Verification items for the finished model (mm, model axes). A direction names the side the tool comes from. Give positions to 0.01 mm unless a question says otherwise; leave off trailing zeros. Order: outer loops, then holes, each group sorted by start corner. A loop starts at its lowest first (then second) coordinate and runs counter-clockwise, first axis right, second up. Notation, with made-up numbers: (20.5, 48.25) - (69.5, 48.25) arc R21 ccw to (69.5, 61.25) - close; hole circle Ø1 at (-10, 52.5). An arc over 180 degrees is marked (long way). Answer as a JSON object with one key per item and string values. Group by question number.
(1) Section check B-B (x = -9.5). Record the boundary of the cut face in (y, z), then the cut area to 3 significant figures.
(2) Access from +Z, -Z, +X, -X, +Y, -Y to the whole of each face (thin tool, end or side, straight path). Record for faces 5 (the face through (-14, 2, 11)), 6 (the face through (-17.859, 62.797, 12.422)).
(3) Mould release check, pull along X, two halves, no side actions. Record for faces 1 (the face through (-1.203, 1.141, 12.422)), 2 (the face through (-5.87, 37.69, 23.51)), 3 (the face through (-19, 32, 12)), 4 (the face through (-8, 4, 0)): +X half, -X half, draft (parallel to the pull), parting line (faces both ways), or undercut.
(4) Section check D-D (y = 51). Record the boundary of the cut face in (x, z).
(5) Thickness scan on line 1 (Y direction, x = -9.5, z = 6.75); line 2 (X direction, y = 20.5, z = 2.5); line 3 (Y direction, x = -9.5, z = 23.3). Record the ranges inside material, lowest first.
(6) Section check A-A (y = 32). Record the boundary of the cut face in (x, z), then the cut area to 3 significant figures.
(7) Section check C-C (z = 20.75). Record the boundary of the cut face in (x, y), then the cut area to 3 significant figures.
```python
from build123d import *

# Parameters (mm, degrees)
F0_W      = 19
F0_H      = 64
F1_DEPTH  = 24.5
F3_DEPTH  = 25
F4_T      = -2
F5_R      = 4
F6_R      = 6.75
F7_DEPTH  = 25
F8_R      = 2
F8_R_2    = 1.25
F9_DEPTH  = 22.5
F10_R     = 6.75
F11_DEPTH = 25


with BuildPart() as f1:
    # F0 (on Top) → F1 (new body)
    with BuildSketch(Plane.XY):
        with Locations((-9.5, 32)):
            Rectangle(F0_W, F0_H)
    extrude(amount=F1_DEPTH)

    # F2 (on face) → F3 (cut)
    with BuildSketch(Plane.YZ):
        with BuildLine():
            Line((21, 0), (43, 0))
            ThreePointArc((43, 0), (32, 11), (21, 0))
        make_face()
    extrude(amount=-F3_DEPTH, mode=Mode.SUBTRACT)

    # F4
    f4_openings = [f1.faces().sort_by_distance(p)[0] for p in [
        (-9.5, 32, 11),
        (-9.5, 10.5, 0),
        (-9.5, 53.5, 0),
    ]]
    offset(amount=F4_T, openings=f4_openings)

    # F5
    f5_edges = [f1.edges().sort_by_distance(p)[0] for p in [
        (0, 0, 12.25),
        (0, 64, 12.25),
        (-19, 64, 12.25),
        (-19, 0, 12.25),
    ]]
    fillet(f5_edges, radius=F5_R)

    # F6 (on face) → F7 (cut)
    with BuildSketch(Plane.XY.offset(24.5)):
        with Locations((-9.5, 32)):
            Circle(F6_R)
    extrude(amount=-F7_DEPTH, mode=Mode.SUBTRACT)

    # F8 (on face) → F9 (join)
    with BuildSketch(Plane(origin=(0, 0, 22.5), x_dir=(1, 0, 0), z_dir=(0, 0, -1))):
        with Locations((-9.5, -3)):
            Circle(F8_R)
        with Locations((-9.5, -3)):
            Circle(F8_R_2, mode=Mode.SUBTRACT)
        with Locations((-9.5, -61)):
            Circle(F8_R)
        with Locations((-9.5, -61)):
            Circle(F8_R_2, mode=Mode.SUBTRACT)
    extrude(amount=F9_DEPTH)

    # F10 (on face) → F11 (cut)
    with BuildSketch(Plane.XY.offset(24.5)):
        with Locations((-9.5, 51)):
            Circle(F10_R)
        with Locations((-9.5, 13)):
            Circle(F10_R)
    extrude(amount=-F11_DEPTH, mode=Mode.SUBTRACT)


solid = f1.part
```
Solutions:
{
 "1": {"outline": "(0, 0) - (2, 0) - (2, 22.5) - (4.25, 22.5) - (4.25, 0) - (5, 0) - (5, 22.5) - (6.25, 22.5) - (6.25, 24.5) - (0, 24.5) - close; (19.75, 22.5) - (25.25, 22.5) - (25.25, 24.5) - (19.75, 24.5) - close; (38.75, 22.5) - (44.25, 22.5) - (44.25, 24.5) - (38.75, 24.5) - close; (57.75, 22.5) - (59, 22.5) - (59, 0) - (59.75, 0) - (59.75, 22.5) - (62, 22.5) - (62, 0) - (64, 0) - (64, 24.5) - (57.75, 24.5) - close", "area": "171 mm2"},
 "2": {"face 5": "-Z", "face 6": "+Z, -Z, -X, +Y"},
 "3": {"face 1": "+X half", "face 2": "undercut", "face 3": "-X half", "face 4": "draft"},
 "4": {"outline": "(-19, 0) - (-17, 0) - (-17, 22.5) - (-16.25, 22.5) - (-16.25, 24.5) - (-19, 24.5) - close; (-2.75, 22.5) - (-2, 22.5) - (-2, 0) - (0, 0) - (0, 24.5) - (-2.75, 24.5) - close"},
 "5": {"line 1": "y = 0 to 2, 4.25 to 5, 59 to 59.75, 62 to 64", "line 2": "x = -19 to -17, -2 to 0", "line 3": "y = 0 to 6.25, 19.75 to 25.25, 38.75 to 44.25, 57.75 to 64"},
 "6": {"outline": "(-19, 11) - (-17, 11) - (-17, 22.5) - (-16.25, 22.5) - (-16.25, 24.5) - (-19, 24.5) - close; (-2.75, 22.5) - (-2, 22.5) - (-2, 11) - (0, 11) - (0, 24.5) - (-2.75, 24.5) - close", "area": "57.0 mm2"},
 "7": {"outline": "(-19, 4) arc R4 ccw to (-15, 0) - (-4, 0) arc R4 ccw to (0, 4) - (0, 60) arc R4 ccw to (-4, 64) - (-15, 64) arc R4 ccw to (-19, 60) - close; hole (-17, 2) - (-11.23, 2) arc R2 cw (long way) to (-7.77, 2) - (-2, 2) - (-2, 62) - (-7.77, 62) arc R2 cw (long way) to (-11.23, 62) - (-17, 62) - close; hole (-10.25, 2) - (-8.75, 2) arc R1.25 ccw (long way) to start; hole (-10.25, 62) arc R1.25 ccw (long way) to (-8.75, 62) - close", "area": "313 mm2"}
}
